For this review, use the dimensioned drawing (mm, ordinates from the lowest corner) and the shaded views. A direction names the side the tool comes from. Round coordinates to 2 decimals unless told otherwise and drop trailing zeros. Write each loop counter-clockwise with the first axis right and the second up, starting at its lowest first coordinate (ties: lowest second). Pieces come first, ordered by that corner, then holes. Notation, with made-up numbers: M -11.75,31 L 2.25,31 A21 cw 2.25,61 Z; hole C 14.5,-22 d2. An arc over 180 degrees is marked long. Use one line per item in the form item = value. Start each with the question number.
Item 1: Add section D-D (y = 16). State the section outline as (x, z) points.
Item 2: Add section C-C (x = 6.5). State the section outline as (y, z) points.
Item 3: Add section A-A (y = 24.75). State the section outline as (x, z) points, and give its area (3 significant figures).
Item 4: For line 1 (Z direction, x = 42, y = 22); line 2 (X direction, y = 26, z = 16.5), list the stretches that pass through material, from the lowest coordinate up. Write a range as [from, to].
Item 5: Add section B-B (x = 15). State the section outline as (y, z) points.
Item 6: For P1, Ø0.9, axis at x = 7, y = 24.5, coming from the +Z side; P2, Ø1.5, axis at y = 17.5, z = 35, coming from the -X side; P3, Ø10, axis at x = 46, y = 18, coming from the +Z side, all flat-tipped, find the tip position at first contact; note any pin that passes through.
Item 7: For the marked faces 1 and 2, list the 3-axis set-ups (+Z, -Z, +X, -X, +Y, -Y) from which the entire face can be reached by the end or side of a thin tool; tool diameter is ignored.
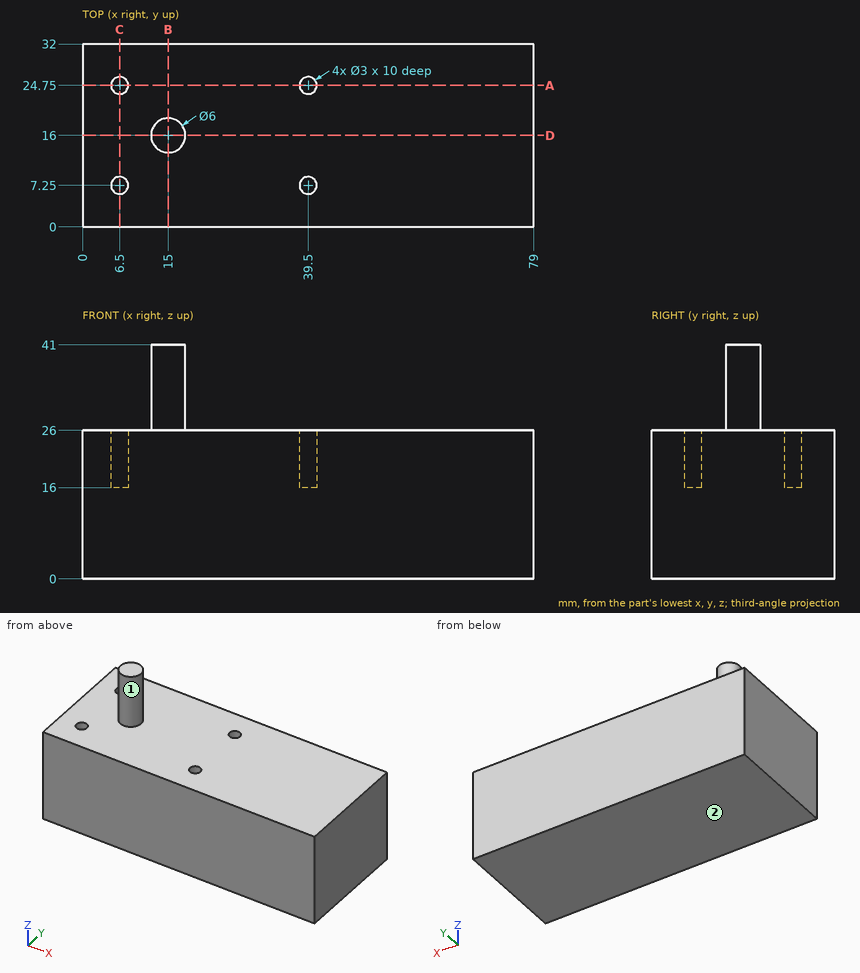
Calculated:
q1.outline = M 0,0 L 79,0 L 79,26 L 18,26 L 18,41 L 12,41 L 12,26 L 0,26 Z
q2.outline = M 0,0 L 32,0 L 32,26 L 26.25,26 L 26.25,16 L 23.25,16 L 23.25,26 L 8.75,26 L 8.75,16 L 5.75,16 L 5.75,26 L 0,26 Z
q3.outline = M 0,0 L 79,0 L 79,26 L 41,26 L 41,16 L 38,16 L 38,26 L 8,26 L 8,16 L 5,16 L 5,26 L 0,26 Z
q3.area = 1,990 mm^2
q4.line_1 = [0, 26]
q4.line_2 = [0, 5.67], [7.33, 38.67], [40.33, 79]
q5.outline = M 0,0 L 32,0 L 32,26 L 19,26 L 19,41 L 13,41 L 13,26 L 0,26 Z
q6.P1 = 16
q6.P2 = 12.1
q6.P3 = 26
q7.face_1 = +Z
q7.face_2 = -Z, +X, -X, +Y, -Y
